The model under review builds one solid part; all positions refer to its coordinate system, in mm. A direction names the side the tool comes from. Coordinates: 2 decimals unless noted, no trailing zeros. Use one line per item in the form item = value. Start each with the question number.
```python
from build123d import *

# Parameters (mm, degrees)
CUT_EXTRUDE1_REACH = 21.23
SKETCH3_R          = 1.5
CUT_EXTRUDE2_DEPTH = 26.95888467
CUT_EXTRUDE3_DEPTH = 10


with BuildPart() as part:
    # Sketch2 → Revolve1 (revolve)
    with BuildSketch(Plane.XY):
        with BuildLine():
            Line((0, 4.5), (11.721248341, 9.383853475))
            Line((11.721248341, 9.383853475), (10.96991248, 15))
            Line((10.96991248, 15), (-10, 22))
            Line((-10, 22), (-10, 23))
            Line((-10, 23), (-9.5, 23))
            add(Edge.make_bspline(
                [(-9.5, 23), (-9.184580705, 24.805210342), (-11.680572374, 29.481442907), (-6.228226752, 39.190854706), (6.249334684, 37.877953806), (13.043419089, 39.508483339), (17.603844738, 30.624473337), (15.729076842, 20)],
                knots=[0, 0, 0, 0, 0.229957765, 0.280779104, 0.508213391, 0.824609493, 1, 1, 1, 1], degree=3))
            Line((15.729076842, 20), (15.729076842, 17))
            Line((15.729076842, 17), (13.729076842, 17))
            Line((13.729076842, 17), (15, 7.5))
            Line((15, 7.5), (9, 5))
            Line((9, 5), (9, 0))
            Line((9, 0), (-1.5, 0))
            Line((-1.5, 0), (-1.5, 4.5))
            Line((-1.5, 4.5), (0, 4.5))
        make_face()
    revolve(axis=Axis((-63.183775164, 0, 0), (1, 0, 0)))

    # Sketch3 → Cut-Extrude1 (cut, up to next)
    with BuildSketch(Plane(origin=(9, 0, 0), x_dir=(0, 0, -1), z_dir=(1, 0, 0)), mode=Mode.PRIVATE) as cut_extrude1_sk1:
        Circle(SKETCH3_R)
    cut_extrude1_tool1 = extrude(cut_extrude1_sk1.sketch, amount=-CUT_EXTRUDE1_REACH, mode=Mode.PRIVATE) & part.part
    add(cut_extrude1_tool1.solids().sort_by_distance((9, 0, 0))[0], mode=Mode.SUBTRACT)

    # Sketch4 → Cut-Extrude2 (cut, through all)
    with BuildSketch(Plane(origin=(15.729076842, 0, 0), x_dir=(0, 0, -1), z_dir=(1, 0, 0))):
        with BuildLine():
            Line((-6.932428082, 12.94427191), (6.932428082, 12.94427191))
            Line((6.932428082, 12.94427191), (7.712767623, 14.018317146))
            ThreePointArc((7.712767623, 14.018317146), (0, 16), (-7.712767623, 14.018317146))
            Line((-7.712767623, 14.018317146), (-6.932428082, 12.94427191))
        make_face()
        with BuildLine():
            Line((-6.932428082, 12.94427191), (-3.237869127, 7.85914776))
            ThreePointArc((-3.237869127, 7.85914776), (0, 8.5), (3.237869127, 7.85914776))
            Line((3.237869127, 7.85914776), (6.932428082, 12.94427191))
            Line((6.932428082, 12.94427191), (-6.932428082, 12.94427191))
        make_face()
        with BuildLine():
            Line((10.168496059, 10.593130901), (14.452972238, -2.593130901))
            Line((14.452972238, -2.593130901), (15.715588138, -3.003379675))
            ThreePointArc((15.715588138, -3.003379675), (15.92873834, -1.508408067), (16, 0))
            ThreePointArc((16, 0), (14.683006668, 6.356832167), (10.9488356, 11.667176137))
            Line((10.9488356, 11.667176137), (10.168496059, 10.593130901))
        make_face()
        with BuildLine():
            Line((8.475050276, -0.650786313), (14.452972238, -2.593130901))
            Line((14.452972238, -2.593130901), (10.168496059, 10.593130901))
            Line((10.168496059, 10.593130901), (6.473937104, 5.508006751))
            ThreePointArc((6.473937104, 5.508006751), (7.977420178, 2.934410896), (8.5, 0))
            ThreePointArc((8.5, 0), (8.493760279, -0.325632198), (8.475050276, -0.650786313))
        make_face()
        with BuildLine():
            Line((13.216904261, -6.397356966), (2, -14.546914944))
            Line((2, -14.546914944), (2, -15.874507866))
            ThreePointArc((2, -15.874507866), (9.404564037, -12.94427191), (14.479520161, -6.807605741))
            Line((14.479520161, -6.807605741), (13.216904261, -6.397356966))
        make_face()
        with BuildLine():
            Line((2, -8.261355821), (2, -14.546914944))
            Line((2, -14.546914944), (13.216904261, -6.397356966))
            Line((13.216904261, -6.397356966), (7.238982298, -4.455012378))
            ThreePointArc((7.238982298, -4.455012378), (4.996174644, -6.876644452), (2, -8.261355821))
        make_face()
        with BuildLine():
            Line((-2, -15.874507866), (-2, -14.546914944))
            Line((-2, -14.546914944), (-13.216904261, -6.397356966))
            Line((-13.216904261, -6.397356966), (-14.479520161, -6.807605741))
            ThreePointArc((-14.479520161, -6.807605741), (-9.404564037, -12.94427191), (-2, -15.874507866))
        make_face()
        with BuildLine():
            Line((-13.216904261, -6.397356966), (-2, -14.546914944))
            Line((-2, -14.546914944), (-2, -8.261355821))
            ThreePointArc((-2, -8.261355821), (-4.996174644, -6.876644452), (-7.238982298, -4.455012378))
            Line((-7.238982298, -4.455012378), (-13.216904261, -6.397356966))
        make_face()
        with BuildLine():
            Line((-15.715588138, -3.003379675), (-14.452972238, -2.593130901))
            Line((-14.452972238, -2.593130901), (-10.168496059, 10.593130901))
            Line((-10.168496059, 10.593130901), (-10.9488356, 11.667176137))
            ThreePointArc((-10.9488356, 11.667176137), (-15.216904261, 4.94427191), (-15.715588138, -3.003379675))
        make_face()
        with BuildLine():
            Line((-10.168496059, 10.593130901), (-14.452972238, -2.593130901))
            Line((-14.452972238, -2.593130901), (-8.475050276, -0.650786313))
            ThreePointArc((-8.475050276, -0.650786313), (-8.083980389, 2.626644452), (-6.473937104, 5.508006751))
            Line((-6.473937104, 5.508006751), (-10.168496059, 10.593130901))
        make_face()
    extrude(amount=-CUT_EXTRUDE2_DEPTH, mode=Mode.SUBTRACT)

    # Sketch5 → Cut-Extrude3 (cut)
    with BuildSketch(Plane.ZY.offset(1.5)):
        Polygon((0, -2.886751346), (2.5, -1.443375673), (2.5, 1.443375673), (0, 2.886751346), (-2.5, 1.443375673), (-2.5, -1.443375673), align=None)
    extrude(amount=-CUT_EXTRUDE3_DEPTH, mode=Mode.SUBTRACT)


solid = part.part
```
1. For P1, Ø5.5, axis at x = 10, y = -12.5, coming from the +Z side; P2, Ø12, axis at y = -6.5, z = 6, coming from the +X side; P3, Ø10, axis at x = -7, y = -9, coming from the +Z side, all flat-tipped, find the tip position at first contact; note any pin that passes through.
2. For L1, parallel to Y at x = 7.25, z = -5.5; L2, parallel to Z at x = 14.65, y = 0; L3, parallel to Z at x = 14.2, y = 0, list the stretches that pass through material, from the lowest coordinate up.
3. Take a section at A-A (x = 1). Count the separate pieces of the cut face and the enclosed holes in it, plus the area to 3 significant figures.
4. For faces 1 (the conical face through (11.34, -3.81, -11.62)), 2 (the cylindrical face through (12.3, 8.5, 0)), 3 (the flat face through (9, -1.2, 1.2)), list the 3-axis set-ups (+Z, -Z, +X, -X, +Y, -Y) from which the entire face can be reached by the end or side of a thin tool; tool diameter is ignored.
Returned:
q1.P1 = 37.11
q1.P2 = 15
q1.P3 = 37.86
q2.L1 = -38.1 to -15.28, -5.13 to 5.13, 15.28 to 38.1
q2.L2 = -35.31 to -17, -8.5 to -7.35, 7.35 to 8.5, 17 to 35.31
q2.L3 = -35.85 to -17, -8.5 to -7.17, 7.17 to 8.5, 17 to 35.85
q3.separate_pieces = 2
q3.enclosed_holes = 2
q3.area = 3,670 mm²
q4.face_1 = -X
q4.face_2 = +X, -X
q4.face_3 = +X
